```python
from build123d import *

# Parameters (mm, degrees)
SKETCH_1_W      = 150
SKETCH_1_H      = 55
SKETCH_1_R      = 1.7
EXTRUDE_1_DEPTH = 2
SKETCH_2_W      = 44
SKETCH_2_H      = 9
EXTRUDE_2_DEPTH = 9


with BuildPart() as part:
    # 草圖1 → 填料-伸長1 (new body)
    with BuildSketch(Plane.XY):
        Rectangle(SKETCH_1_W, SKETCH_1_H)
        with Locations((-72, 24.5)):
            Circle(SKETCH_1_R, mode=Mode.SUBTRACT)
        with Locations(Location((72, 24.5, 0), (0, 0, 180))):
            Circle(SKETCH_1_R, mode=Mode.SUBTRACT)
        with Locations((72, -24.5)):
            Circle(SKETCH_1_R, mode=Mode.SUBTRACT)
        with Locations(Location((-72, -24.5, 0), (0, 0, 180))):
            Circle(SKETCH_1_R, mode=Mode.SUBTRACT)
    extrude(amount=EXTRUDE_1_DEPTH)

    # 草圖2 → 填料-伸長2 (add)
    with BuildSketch(Plane.XY.offset(2)):
        with Locations((8, 1)):
            Rectangle(SKETCH_2_W, SKETCH_2_H)
    extrude(amount=EXTRUDE_2_DEPTH)


solid = part.part
```
Part model, mm, in its own coordinate system. A direction names the side the tool comes from. Round coordinates to 2 decimals unless told otherwise and drop trailing zeros. Loops run counter-clockwise (first coordinate to the right, second up) from the corner with the lowest first, then second, coordinate; pieces in that order, holes last.
Item 1: 3-axis set-ups, long thin cutter, end or side, ignore diameter. For faces 1 (the face through (-1, 0, 0)), 2 (the face through (8, 5.5, 6)), 3 (the face through (30, 1, 6)): which of +Z, -Z, +X, -X, +Y, -Y reach the whole face in a straight line?
Item 2: Mould opens along Y. For faces 4 (the face through (8, -3.5, 6)), 5 (the face through (-14, 1, 6)), 6 (the face through (-70.3, -24.57, 0.99)) say: +Y half, -Y half, draft (parallel to the pull), parting line (faces both ways), or undercut.
Item 3: Cut at C-C, the plane x = 15. Give the cut face in (y, z).
Item 4: Drill centre lines: line 1 (Y direction, x = -72, z = 1.5); line 2 (Z direction, x = 37, y = -10); line 3 (Y direction, x = -4, z = 5.75). Where is each one in solid material? Low to high.
Item 5: Cut at B-B, the plane x = 72. Give the cut face in (y, z), then the cut area to 3 significant figures.
Item 6: Cut at A-A, the plane y = 24.5. Give the cut face in (x, z), then the cut area to 3 significant figures.
Item 7: Drop flat-ended pins along their axis: P1, Ø4, axis at x = -10.5, y = -22, coming from the -Z side; P2, Ø4, axis at x = -29.5, y = -4, coming from the +Z side; P3, Ø6, axis at y = -6, z = 7.5, coming from the +X side; P4, Ø4.5, axis at x = 0.5, z = 4.5, coming from the +Y side. Give the stop position or say it passes through.
Item 8: Cut at D-D, the plane y = 0. Give the cut face in (x, z), then the cut area to 3 significant figures.
A:
1. face 1: -Z, +X, -X, +Y, -Y
1. face 2: +Z, +X, -X, +Y
1. face 3: +Z, +X, +Y, -Y
2. face 4: -Y half
2. face 5: draft
2. face 6: undercut
3. outline: (-27.5, 0) - (27.5, 0) - (27.5, 2) - (5.5, 2) - (5.5, 11) - (-3.5, 11) - (-3.5, 2) - (-27.5, 2) - close
4. line 1: y = -27.5 to -26.2, -22.8 to 22.8, 26.2 to 27.5
4. line 2: z = 0 to 2
4. line 3: y = -3.5 to 5.5
5. outline: (-27.5, 0) - (-26.2, 0) - (-26.2, 2) - (-27.5, 2) - close; (-22.8, 0) - (22.8, 0) - (22.8, 2) - (-22.8, 2) - close; (26.2, 0) - (27.5, 0) - (27.5, 2) - (26.2, 2) - close
5. area: 96.4 mm2
6. outline: (-75, 0) - (-73.7, 0) - (-73.7, 2) - (-75, 2) - close; (-70.3, 0) - (70.3, 0) - (70.3, 2) - (-70.3, 2) - close; (73.7, 0) - (75, 0) - (75, 2) - (73.7, 2) - close
6. area: 286 mm2
7. P1: stops at z = 0
7. P2: stops at z = 2
7. P3: stops at x = 30
7. P4: stops at y = 5.5
8. outline: (-75, 0) - (75, 0) - (75, 2) - (30, 2) - (30, 11) - (-14, 11) - (-14, 2) - (-75, 2) - close
8. area: 696 mm2
